Design review of the part built by this model. Coordinates are the model's own, in mm. A direction names the side the tool comes from. Coordinates: 2 decimals unless noted, no trailing zeros.
from build123d import *

# Parameters (mm, degrees)
F1_DEPTH = 25


# Not quite as in the source:
# - ends of sketch curves that miss each other by under 0.0002 mm in the source are joined


with BuildPart() as f1:
    # F0 (on Front) → F1 (new body)
    with BuildSketch(Plane.XZ):
        with BuildLine():
            ThreePointArc((-12.0672760652, 8.9096491574), (-11.3814883912, 8.9771930389), (-10.7737513132, 8.6523506868))
            Line((-10.7737513132, 8.6523506868), (-6, 3.8786))
            Line((-6, 3.8786), (-6, 0.5))
            Line((-6, 0.5), (-5.5, 0))
            Line((-5.5, 0), (-6, -0.5))
            Line((-6, -0.5), (-6, -3.8786))
            Line((-6, -3.8786), (-10.7738, -8.6524))
            ThreePointArc((-10.7738, -8.6524), (-11.3814883912, -8.9771930389), (-12.0672760652, -8.9096491574))
            ThreePointArc((-12.0672760652, -8.9096491574), (-12.5999492171, -8.4725051968), (-12.799999999, -7.8131))
            Line((-12.799999999, -7.8131), (-12.8, -4))
            Line((-12.8, -4), (-14.5, -4))
            Line((-14.5, -4), (-15, -4.5))
            Line((-15, -4.5), (-15, -9.5))
            Line((-15, -9.5), (-14.5, -10))
            Line((-14.5, -10), (-15, -10.5))
            Line((-15, -10.5), (-15, -13))
            ThreePointArc((-15, -13), (-14.4141844722, -14.4142216524), (-13, -15.0000239995))
            Line((-13, -15.0000239995), (-10.5, -15))
            Line((-10.5, -15), (-10, -14.5))
            Line((-10, -14.5), (-9.5, -15))
            Line((-9.5, -15), (-4.5, -15))
            Line((-4.5, -15), (-4, -14.5))
            Line((-4, -14.5), (-4, -12.8))
            Line((-4, -12.8), (-7.8131, -12.8))
            ThreePointArc((-7.8131, -12.8), (-8.4725048128, -12.5999494737), (-8.9096488038, -12.0672769187))
            ThreePointArc((-8.9096488038, -12.0672769187), (-8.977199798, -11.3815223738), (-8.6523996854, -10.7738003146))
            Line((-8.6523996854, -10.7738003146), (-3.8786, -6))
            Line((-3.8786, -6), (-0.5, -6))
            Line((-0.5, -6), (0, -5.5))
            Line((0, -5.5), (0.5, -6))
            Line((0.5, -6), (3.8786, -6))
            Line((3.8786, -6), (8.6524, -10.7738))
            ThreePointArc((8.6524, -10.7738), (8.977199798, -11.3815223738), (8.9096491574, -12.0672760652))
            ThreePointArc((8.9096491574, -12.0672760652), (8.4725048128, -12.5999494737), (7.8131, -12.799999999))
            Line((7.8131, -12.799999999), (4, -12.8))
            Line((4, -12.8), (4, -14.5))
            Line((4, -14.5), (4.5, -15))
            Line((4.5, -15), (9.5, -15))
            Line((9.5, -15), (10, -14.5))
            Line((10, -14.5), (10.5, -15))
            Line((10.5, -15), (13, -15))
            ThreePointArc((13, -15), (14.4141844722, -14.4142216524), (14.999955, -13.000024))
            Line((14.999955, -13.000024), (15, -10.5))
            Line((15, -10.5), (14.5, -10))
            Line((14.5, -10), (15, -9.5))
            Line((15, -9.5), (15, -4.5))
            Line((15, -4.5), (14.5, -4))
            Line((14.5, -4), (12.8, -4))
            Line((12.8, -4), (12.8, -7.8131))
            ThreePointArc((12.8, -7.8131), (12.5999492171, -8.4725051968), (12.0672760652, -8.9096491574))
            ThreePointArc((12.0672760652, -8.9096491574), (11.3814883912, -8.9771930389), (10.7737513132, -8.6523506868))
            Line((10.7737513132, -8.6523506868), (6, -3.8786))
            Line((6, -3.8786), (6, -0.5))
            Line((6, -0.5), (5.5, 0))
            Line((5.5, 0), (6, 0.5))
            Line((6, 0.5), (6, 3.8786))
            Line((6, 3.8786), (10.7738, 8.6524))
            ThreePointArc((10.7738, 8.6524), (11.3814883912, 8.9771930389), (12.0672760652, 8.9096491574))
            ThreePointArc((12.0672760652, 8.9096491574), (12.5999492171, 8.4725051968), (12.799999999, 7.8131))
            Line((12.799999999, 7.8131), (12.8, 4))
            Line((12.8, 4), (14.5, 4))
            Line((14.5, 4), (15, 4.5))
            Line((15, 4.5), (15, 9.5))
            Line((15, 9.5), (14.5, 10))
            Line((14.5, 10), (15, 10.5))
            Line((15, 10.5), (15, 13))
            ThreePointArc((15, 13), (14.4141844722, 14.4142216524), (13, 15.0000239995))
            Line((13, 15.0000239995), (10.5, 15))
            Line((10.5, 15), (10, 14.5))
            Line((10, 14.5), (9.5, 15))
            Line((9.5, 15), (4.5, 15))
            Line((4.5, 15), (4, 14.5))
            Line((4, 14.5), (4, 12.8))
            Line((4, 12.8), (7.8131, 12.8))
            ThreePointArc((7.8131, 12.8), (8.4725048128, 12.5999494737), (8.9096488038, 12.0672769187))
            ThreePointArc((8.9096488038, 12.0672769187), (8.977199798, 11.3815223738), (8.6523996854, 10.7738003146))
            Line((8.6523996854, 10.7738003146), (3.8786, 6))
            Line((3.8786, 6), (0.5, 6))
            Line((0.5, 6), (0, 5.5))
            Line((0, 5.5), (-0.5, 6))
            Line((-0.5, 6), (-3.8786, 6))
            Line((-3.8786, 6), (-8.6524, 10.7738))
            ThreePointArc((-8.6524, 10.7738), (-8.977199798, 11.3815223738), (-8.9096491574, 12.0672760652))
            ThreePointArc((-8.9096491574, 12.0672760652), (-8.4725048128, 12.5999494737), (-7.8131, 12.799999999))
            Line((-7.8131, 12.799999999), (-4, 12.8))
            Line((-4, 12.8), (-4, 14.5))
            Line((-4, 14.5), (-4.5, 15))
            Line((-4.5, 15), (-9.5, 15))
            Line((-9.5, 15), (-10, 14.5))
            Line((-10, 14.5), (-10.5, 15))
            Line((-10.5, 15), (-13, 15))
            ThreePointArc((-13, 15), (-14.4141844722, 14.4142216524), (-14.999955, 13.000024))
            Line((-14.999955, 13.000024), (-15, 10.5))
            Line((-15, 10.5), (-14.5, 10))
            Line((-14.5, 10), (-15, 9.5))
            Line((-15, 9.5), (-15, 4.5))
            Line((-15, 4.5), (-14.5, 4))
            Line((-14.5, 4), (-12.8, 4))
            Line((-12.8, 4), (-12.8, 7.8131))
            ThreePointArc((-12.8, 7.8131), (-12.5999492171, 8.4725051968), (-12.0672760652, 8.9096491574))
        make_face()
        with BuildLine():
            Line((-4.2426, -3.182), (-2.8752, -1.8146))
            ThreePointArc((-2.8752, -1.8146), (-3.4, 0), (-2.8752481958, 1.8146481236))
            Line((-2.8752481958, 1.8146481236), (-4.2426, 3.182))
            Line((-4.2426, 3.182), (-3.182, 4.2426))
            Line((-3.182, 4.2426), (-1.8146, 2.8752))
            ThreePointArc((-1.8146, 2.8752), (0, 3.4), (1.8146481236, 2.8752481958))
            Line((1.8146481236, 2.8752481958), (3.182, 4.2426))
            Line((3.182, 4.2426), (4.2426, 3.182))
            Line((4.2426, 3.182), (2.8752, 1.8146))
            ThreePointArc((2.8752, 1.8146), (3.4, 0), (2.8752481958, -1.8146481236))
            Line((2.8752481958, -1.8146481236), (4.2426, -3.182))
            Line((4.2426, -3.182), (3.182, -4.2426))
            Line((3.182, -4.2426), (1.8146, -2.8752))
            ThreePointArc((1.8146, -2.8752), (0, -3.4), (-1.8146481236, -2.8752481958))
            Line((-1.8146481236, -2.8752481958), (-3.182, -4.2426))
            Line((-3.182, -4.2426), (-4.2426, -3.182))
        make_face(mode=Mode.SUBTRACT)
    extrude(amount=F1_DEPTH)


solid = f1.part
Q1. The part is to be moulded in two halves that separate along Z. For faces 5 (the flat face through (15, -12, 7)), 6 (the cylindrical face through (0, -12.3, 3.4)), 7 (the flat face through (-7, -12, -15)), say which applies: pulls with the +Z half, pulls with the -Z half, needs draft (parallel to the pull), parting line crosses it, or undercut.
Q2. For line 1 (X direction, y = -22.5, z = 7.5); line 2 (X direction, y = -21.25, z = 11.5); line 3 (X direction, y = -21, z = -8), list the stretches that pass through material, from the lowest coordinate up.
Q3. Machinability: for faces 1 (the flat face through (-3.57, -12.32, -2.51)), 2 (the flat face through (4, -12, 14)), 3 (the flat face through (14, -12, -4)), 4 (the flat face through (-14, -12, 4)), which of the approach directions +Z, -Z, +X, -X, +Y, -Y give a long, thin tool a straight path to every point of the face, cutting with its end or side? Answer none if there is none.
Q4. Clearance check with flat-ended pins moving along their axes: pin 1 Ø1 at (x, y) = (-2.5, -16.5) entering from +Z; pin 2 Ø3.5 at (y, z) = (-7, -1.5) entering from -X; pin 3 Ø0.5 at (x, y) = (-13.5, -9) entering from -Z. State where each tip first meets the part, or that it passes through.
Entries:
1. face 5: needs draft
1. face 6: undercut
1. face 7: pulls with the -Z half
2. line 1: x = -15 to -12.8, -9.62 to -5.38, 5.38 to 9.62, 12.8 to 15
2. line 2: x = -15 to -8.99, 8.99 to 15
2. line 3: x = -15 to -12.79, -10.12 to -5.88, 5.88 to 10.12, 12.79 to 15
3. face 1: +Y, -Y
3. face 2: +Z, +Y, -Y
3. face 3: +X, +Y, -Y
3. face 4: -X, +Y, -Y
4. pin 1: stops at z = 6
4. pin 2: stops at x = -6
4. pin 3: stops at z = -14.98
